Could you check a few things on this model? Use its own coordinates, in mm. A direction names the side the tool comes from. Give positions to 0.01 mm unless a question says otherwise; leave off trailing zeros. Order: outer loops, then holes, each group sorted by start corner. A loop starts at its lowest first (then second) coordinate and runs counter-clockwise, first axis right, second up. Notation, with made-up numbers: (18.5, 60.25) -> (64.5, 60.25) arc R23 cw to (64.5, 82.25) -> close; hole circle Ø4 at (81.25, -2.5). An arc over 180 degrees is marked (long way). Answer as CSV lines item,"result". Start each with the question number.
(1) I want a section at D-D (x = 2.25). Please give me the cut outline in (y, z).
(2) On a 3-axis mill with a long thin cutter (end or side, diameter ignored), from which of +Z, -Z, +X, -X, +Y, -Y can I reach the whole of each face in a straight line? I mean faces 1 (the face through (-2.2, -2.683, 18.9)), 2 (the face through (0, -3, 24)), 3 (the face through (-0.7, -1, 7)), 4 (the face through (-3.49, 2.51, 6.9)), 5 (the face through (0, -3, 21)). Say none if no direction works.
(3) I need wall thicknesses on L1, parallel to Z at x = 0, y = -2.85; L2, parallel to X at y = -1.5, z = 8.25; L3, parallel to X at y = 1.5, z = 12.25. Which ranges of each line are inside material? Lowest first, please.
(4) Will these pins go through, and if not, where does the flat tip stop? pin 1 Ø2.5 at (x, z) = (0, 19) entering from +Y (3 decimals); pin 2 Ø2.5 at (x, z) = (1, 5) entering from +Y; pin 3 Ø3 at (x, z) = (-1.5, 17.5) entering from +Y.
(5) I want a section at A-A (y = 0.5). Please give me the cut outline in (x, z), plus the area to 3 significant figures.
(6) I want a section at C-C (z = 19). Please give me the cut outline in (x, y).
(7) We'd pull the mould along X, two halves only. Please class faces 6 (the face through (3.465, 2.522, 6.902)), 7 (the face through (-1, -1.683, 7)), 8 (the face through (0, -1, 14)), 9 (the face through (4.85, 0, 6)): released by +X, released by -X, zero draft, split by the parting line, or undercut.
(8) I want a section at B-B (x = 0). Please give me the cut outline in (y, z).
```python
from build123d import *

# Parameters (mm, degrees)
PAD_DEPTH    = 14
SKETCH001_W  = 9.7
SKETCH001_H  = 1
PAD001_DEPTH = 10
SKETCH002_R  = 2
POCKET_DEPTH = 5


with BuildPart() as part:
    # Sketch → Pad (new body)
    with BuildSketch(Plane.XY):
        Polygon((-2.75, 3.516621), (-4.85, 3.516621), (-4.85, -3.683379), (4.85, -3.683379), (4.85, 3.516621), (2.75, 3.516621), (2.75, 2.916621), (4.2, 2.116621), (4.2, -0.683379), (-0.7, -0.683379), (-0.7, -1.683379), (-1.9, -1.683379), (-1.9, -0.683379), (-4.2, -0.683379), (-4.2, 2.116621), (-2.75, 2.916621), align=None)
    extrude(amount=PAD_DEPTH)

    # Sketch001 → Pad001 (new body)
    with BuildSketch(Plane.XY.offset(14)):
        with Locations((0, -3.183379)):
            Rectangle(SKETCH001_W, SKETCH001_H)
    extrude(amount=PAD001_DEPTH)

    # Sketch002 → Pocket (cut)
    with BuildSketch(Plane(origin=(0, -2.683379, 0), x_dir=(-1, 0, 0), z_dir=(0, 1, 0))):
        with Locations((0, 19)):
            Circle(SKETCH002_R)
    extrude(amount=-POCKET_DEPTH, mode=Mode.SUBTRACT)


solid = part.part
```
Final values:
1,outline,"(-3.68, 0) -> (-0.68, 0) -> (-0.68, 14) -> (-2.68, 14) -> (-2.68, 24) -> (-3.68, 24) -> close"
2,face 1,"+Z, +X, -X, +Y"
2,face 2,"+Z, +X, -X, +Y, -Y"
2,face 3,"+Z, -Z, +Y"
2,face 4,"+Z, -Z"
2,face 5,"+Y, -Y"
3,L1,"0 to 17, 21 to 24"
3,L2,"-4.85 to -1.9, -0.7 to 4.85"
3,L3,"-4.85 to -4.2, 4.2 to 4.85"
4,pin 1,"through"
4,pin 2,"y = -0.68"
4,pin 3,"y = -2.68"
5,outline,"(-4.85, 0) -> (-4.2, 0) -> (-4.2, 14) -> (-4.85, 14) -> close; (4.2, 0) -> (4.85, 0) -> (4.85, 14) -> (4.2, 14) -> close"
5,area,"18.2 mm²"
6,outline,"(-4.85, -3.68) -> (-2, -3.68) -> (-2, -2.68) -> (-4.85, -2.68) -> close; (2, -3.68) -> (4.85, -3.68) -> (4.85, -2.68) -> (2, -2.68) -> close"
7,face 6,"undercut"
7,face 7,"undercut"
7,face 8,"zero draft"
7,face 9,"released by +X"
8,outline,"(-3.68, 0) -> (-0.68, 0) -> (-0.68, 14) -> (-2.68, 14) -> (-2.68, 17) -> (-3.68, 17) -> close; (-3.68, 21) -> (-2.68, 21) -> (-2.68, 24) -> (-3.68, 24) -> close"
